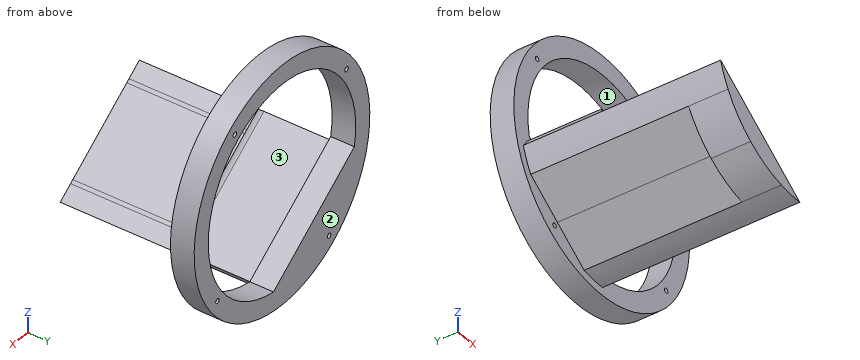
from build123d import *

# Parameters (mm, degrees)
SKETCH2_R           = 75.63
BOSS_EXTRUDE1_DEPTH = 15
SKETCH5_R           = 63.5
CUT_EXTRUDE1_DEPTH  = 109.003674937
BOSS_EXTRUDE2_START = -15
BOSS_EXTRUDE2_DEPTH = 15
BOSS_EXTRUDE3_DEPTH = 125
CUT_EXTRUDE4_DEPTH  = 100
SKETCH7_R           = 1.5
CUT_EXTRUDE2_DEPTH  = 15
SKETCH8_W           = 84.415638362
SKETCH8_H           = 49.5
BOSS_EXTRUDE4_DEPTH = 6
FILLET1_R           = 6


with BuildPart() as part:
    # Sketch2 → Boss-Extrude1 (new body)
    with BuildSketch(Plane(origin=(0, 0, 0), x_dir=(1, 0, 0), z_dir=(0, 1, 0))):
        with Locations(Location((0, 0, 0), (0, 0, 270))):
            Circle(SKETCH2_R)
    extrude(amount=BOSS_EXTRUDE1_DEPTH)

    # Sketch5 → Cut-Extrude1 (cut, through all)
    with BuildSketch(Plane(origin=(0, 15, 0), x_dir=(1, 0, 0), z_dir=(0, 1, 0))):
        with Locations(Location((0, 0, 0), (0, 0, 270))):
            Circle(SKETCH5_R)
    extrude(amount=-CUT_EXTRUDE1_DEPTH, mode=Mode.SUBTRACT)

    # Sketch6 → Boss-Extrude2 (add)
    with BuildSketch(Plane.XZ.offset(BOSS_EXTRUDE2_START)):
        with BuildLine():
            Line((7.313069509, -63.077484211), (-62.311802931, -12.226578243))
            ThreePointArc((-62.311802931, -12.226578243), (-37.452220614, -51.279441993), (7.313069509, -63.077484211))
        make_face()
    extrude(amount=BOSS_EXTRUDE2_DEPTH)

    # Sketch6<5> → Boss-Extrude3 (add)
    with BuildSketch(Plane.XZ):
        with BuildLine():
            Line((-8.246344057, -64.096711575), (-10.190161052, -62.677034213))
            ThreePointArc((-10.190161052, -62.677034213), (-37.452220614, -51.279441993), (-56.604547366, -28.778033593))
            Line((-56.604547366, -28.778033593), (-58.548364361, -27.358356231))
            ThreePointArc((-58.548364361, -27.358356231), (-49.90104688, -41.064292825), (-38.115744208, -52.187936044))
            ThreePointArc((-38.115744208, -52.187936044), (-23.933565149, -60.029784976), (-8.246344057, -64.096711575))
        make_face()
        with BuildLine():
            Line((0.687581465, -70.621652889), (-8.246344057, -64.096711575))
            ThreePointArc((-8.246344057, -64.096711575), (-23.933565149, -60.029784976), (-38.115744208, -52.187936044))
            Line((-38.115744208, -52.187936044), (-15.111189696, -68.989438112))
            ThreePointArc((-15.111189696, -68.989438112), (-7.25783369, -70.251081665), (0.687581465, -70.621652889))
        make_face()
        with BuildLine():
            Line((-61.120298719, -35.386433976), (-38.115744208, -52.187936044))
            ThreePointArc((-38.115744208, -52.187936044), (-49.90104688, -41.064292825), (-58.548364361, -27.358356231))
            Line((-58.548364361, -27.358356231), (-67.482289883, -20.833414917))
            ThreePointArc((-67.482289883, -20.833414917), (-64.711699404, -28.289336954), (-61.120298719, -35.386433976))
        make_face()
        with BuildLine():
            Line((-15.111189696, -68.989438112), (-38.115744208, -52.187936044))
            Line((-38.115744208, -52.187936044), (-41.654536706, -57.033237649))
            ThreePointArc((-41.654536706, -57.033237649), (-29.005596113, -64.393835257), (-15.111189696, -68.989438112))
        make_face()
        with BuildLine():
            Line((-41.654536706, -57.033237649), (-38.115744208, -52.187936044))
            Line((-38.115744208, -52.187936044), (-61.120298719, -35.386433976))
            ThreePointArc((-61.120298719, -35.386433976), (-52.514881, -47.223700602), (-41.654536706, -57.033237649))
        make_face()
        with BuildLine():
            ThreePointArc((-56.604547366, -28.778033593), (-37.452220614, -51.279441993), (-10.190161052, -62.677034213))
            Line((-10.190161052, -62.677034213), (-33.397354209, -45.727533903))
            Line((-33.397354209, -45.727533903), (-56.604547366, -28.778033593))
        make_face()
    extrude(amount=BOSS_EXTRUDE3_DEPTH)

    # Sketch6<14> → Cut-Extrude4 (cut)
    with BuildSketch(Plane.XZ):
        with BuildLine():
            Line((-15.111189696, -68.989438112), (-38.115744208, -52.187936044))
            Line((-38.115744208, -52.187936044), (-41.654536706, -57.033237649))
            ThreePointArc((-41.654536706, -57.033237649), (-29.005596113, -64.393835257), (-15.111189696, -68.989438112))
        make_face()
        with BuildLine():
            Line((-41.654536706, -57.033237649), (-38.115744208, -52.187936044))
            Line((-38.115744208, -52.187936044), (-61.120298719, -35.386433976))
            ThreePointArc((-61.120298719, -35.386433976), (-52.514881, -47.223700602), (-41.654536706, -57.033237649))
        make_face()
    extrude(amount=CUT_EXTRUDE4_DEPTH, mode=Mode.SUBTRACT)

    # Sketch7 → Cut-Extrude2 (cut)
    with BuildSketch(Plane(origin=(0, 15, 0), x_dir=(1, 0, 0), z_dir=(0, 1, 0))):
        with Locations(Location((40.592898957, -55.579647168, 0), (0, 0, 270))):
            Circle(SKETCH7_R)
        with Locations(Location((-55.579647168, -40.592898957, 0), (0, 0, 270))):
            Circle(SKETCH7_R)
        with Locations(Location((-40.592898957, 55.579647168, 0), (0, 0, 270))):
            Circle(SKETCH7_R)
        with Locations(Location((55.579647168, 40.592898957, 0), (0, 0, 270))):
            Circle(SKETCH7_R)
    extrude(amount=-CUT_EXTRUDE2_DEPTH, mode=Mode.SUBTRACT)

    # Sketch8 → Boss-Extrude4 (add)
    with BuildSketch(Plane(origin=(-33.397354209, 0, -45.727533903), x_dir=(0.8075502676015422, 0, -0.5897987498263095), z_dir=(0.5897987498263095, 0, 0.8075502676015424))):
        with Locations((0, -24.75)):
            Rectangle(SKETCH8_W, SKETCH8_H)
    extrude(amount=BOSS_EXTRUDE4_DEPTH)

    # Fillet1
    fillet1_edges = [part.edges().sort_by_distance(p)[0] for p in [
        (-29.85856171, -49.5, -40.882232297),
    ]]
    fillet(fillet1_edges, radius=FILLET1_R - 0.0001)  # a hair under: the kernel refuses the full size


solid = part.part
Verification items for the finished model (mm, model axes). Face numbers are marked on the shaded views. Round coordinates to 2 decimals unless told otherwise and drop trailing zeros. Loops run counter-clockwise (first coordinate to the right, second up) from the corner with the lowest first, then second, coordinate; pieces in that order, holes last. Notation, with made-up numbers: (-21, 1) - (33, 1) arc R12 ccw to (33, 5) - close; hole circle Ø10 at (83, 6.5). An arc over 180 degrees is marked (long way). Answer in a Markdown table with one row per item. Add a question column.
Q1. Gauge pin test, flat ends, axial feed: pin 1 (10 mm diameter, centred on y = -62, z = -39.5, fed in from -X) (3 decimals); pin 2 (10 mm diameter, centred on y = -93.5, z = -36.5, fed in from +X); pin 3 (15 mm diameter, centred on x = -28.5, z = -46.5, fed in from -Y); pin 4 (1.5 mm diameter, centred on x = -37.5, y = -97, fed in from -Z). Record the tip position at first contact, or that the pin passes through.
Q2. Release check for a two-part mould opening along X. For the marked faces 1, 2 and 3 record: pulls with the +X half, pulls with the -X half, needs draft (parallel to the pull), parting line crosses it, or undercut.
Q3. Material ranges on line 1 (Y direction, x = -8.5, z = -53); line 2 (X direction, y = 8.5, z = -39); line 3 (X direction, y = 8.5, z = -46) (3 decimals), recorded low to high.
Q4. Section check A-A on z = 0. Enter the section's corners in (x, y), plus the area to 3 significant figures.
Q5. Section check D-D on y = -69. Enter the section's corners in (x, z) (3 decimals).
Q6. Section check C-C on x = 21.5. Enter the section's corners in (y, z).
Found:
| question | item | result |
|---|---|---|
| 1 | pin 1 | stops at x = -61.625 |
| 1 | pin 2 | stops at x = -39.19 |
| 1 | pin 3 | stops at y = -125 |
| 1 | pin 4 | stops at z = -53.19 |
| 2 | face 1 | undercut |
| 2 | face 2 | needs draft |
| 2 | face 3 | pulls with the +X half |
| 3 | line 1 | y = 0 to 15 |
| 3 | line 2 | x = -64.8 to -25.65, 50.11 to 64.8 |
| 3 | line 3 | x = -60.032 to -16.069, 43.775 to 60.032 |
| 4 | outline | (-75.63, 0) - (-63.5, 0) - (-63.5, 15) - (-75.63, 15) - close; (63.5, 0) - (75.63, 0) - (75.63, 15) - (63.5, 15) - close |
| 4 | area | 364 mm² |
| 5 | outline | (-67.482, -20.833) arc R70.625 ccw to (-61.12, -35.386) - (-15.111, -68.989) arc R70.625 ccw to (0.688, -70.622) - close |
| 6 | outline | (0, -72.51) - (15, -72.51) - (15, -59.75) - (0, -59.75) - close; (0, 59.75) - (15, 59.75) - (15, 72.51) - (0, 72.51) - close |
